```python
from build123d import *

# Parameters (mm, degrees)
F0_W     = 127
F0_H     = 10.16
F1_DEPTH = 10.16
F2_R     = 5.07999
F3_R     = 2.54
F4_DEPTH = 25.4


# Not quite as in the source:
# - a fillet or chamfer is up to 0.001 mm smaller than in the source, because OpenCascade refuses the exact size
# - a pattern or mirror of a feature is missing from the dataset's text; its kind, count and spacing are read off the source's solid


with BuildPart() as f1:
    # F0 (on Top) → F1 (new body)
    with BuildSketch(Plane.XY):
        Rectangle(F0_W, F0_H)
    extrude(amount=F1_DEPTH)

    # F2 (radius 5.08 in the source; OpenCascade refuses exactly that, so slightly less here)
    f2_edges = [f1.edges().sort_by_distance(p)[0] for p in [
        (-63.5, -5.08, 5.08),
        (-63.5, 5.08, 5.08),
        (63.5, -5.08, 5.08),
        (63.5, 5.08, 5.08),
    ]]
    fillet(f2_edges, radius=F2_R)

    # F3 (on face) → F4 (cut)
    with BuildSketch(Plane(origin=(0, 0, 0), x_dir=(1, 0, 0), z_dir=(0, 0, -1))):
        with Locations((-58.42, 0)):
            Circle(F3_R)
    f4 = extrude(amount=-F4_DEPTH, mode=Mode.SUBTRACT)

    # F4_copies: F4 across plane
    add(f4.mirror(Plane(origin=(0, 0, 0), x_dir=(0, 0, 1), z_dir=(1, 0, 0))), mode=Mode.SUBTRACT)


solid = f1.part
```
Could you check a few things on this model? Use its own coordinates, in mm. Round coordinates to 2 decimals unless told otherwise and drop trailing zeros. Loops run counter-clockwise (first coordinate to the right, second up) from the corner with the lowest first, then second, coordinate; pieces in that order, holes last.
Q1. I want a section at B-B (y = -1.5). Write out the boundary of the cut face in (x, z), and give its area (3 significant figures).
Q2. For P1, Ø3, axis at y = 2.5, z = 4.5, coming from the -X side; P2, Ø2, axis at y = 3, z = 2, coming from the -X side, each with a flat end and sliding along its axis, tell me the tip position at first contact or that it passes through.
Q3. Please list where these lines run through material, in increasing order: L1, parallel to X at y = 0, z = 8; L2, parallel to X at y = -2.25, z = 5.25; L3, parallel to Y at x = -58.42, z = 4.5.
Q4. Thinking about a two-plate mould opening in Y: for faces 1 (the flat face through (-1, 0, 0)), 2 (the flat face through (-1, 5.08, 5)), 3 (the cylindrical face through (-60.958, -0.112, 5.009)), 4 (the cylindrical face through (60.958, -0.112, 5.009)), which applies, pulls with the +Y half, pulls with the -Y half, needs draft (parallel to the pull), parting line crosses it, or undercut?
Q5. I want a section at A-A (z = 4.5). Give the number of separate pieces and of enclosed holes in the cut face, and give its area (3 significant figures).
Answer below:
1. outline: (-63.27, 0) - (-60.47, 0) - (-60.47, 10.16) - (-63.27, 10.16) - close; (-56.37, 0) - (56.37, 0) - (56.37, 10.16) - (-56.37, 10.16) - close; (60.47, 0) - (63.27, 0) - (63.27, 10.16) - (60.47, 10.16) - close
1. area: 1,200 mm2
2. P1: stops at x = -63.4
2. P2: stops at x = -63.09
3. L1: x = -63.5 to -60.96, -55.88 to 55.88, 60.96 to 63.5
3. L2: x = -62.97 to -59.6, -57.24 to 57.24, 59.6 to 62.97
3. L3: y = -5.08 to -2.54, 2.54 to 5.08
4. face 1: needs draft
4. face 2: pulls with the +Y half
4. face 3: undercut
4. face 4: undercut
5. separate pieces: 1
5. enclosed holes: 2
5. area: 1,230 mm2
